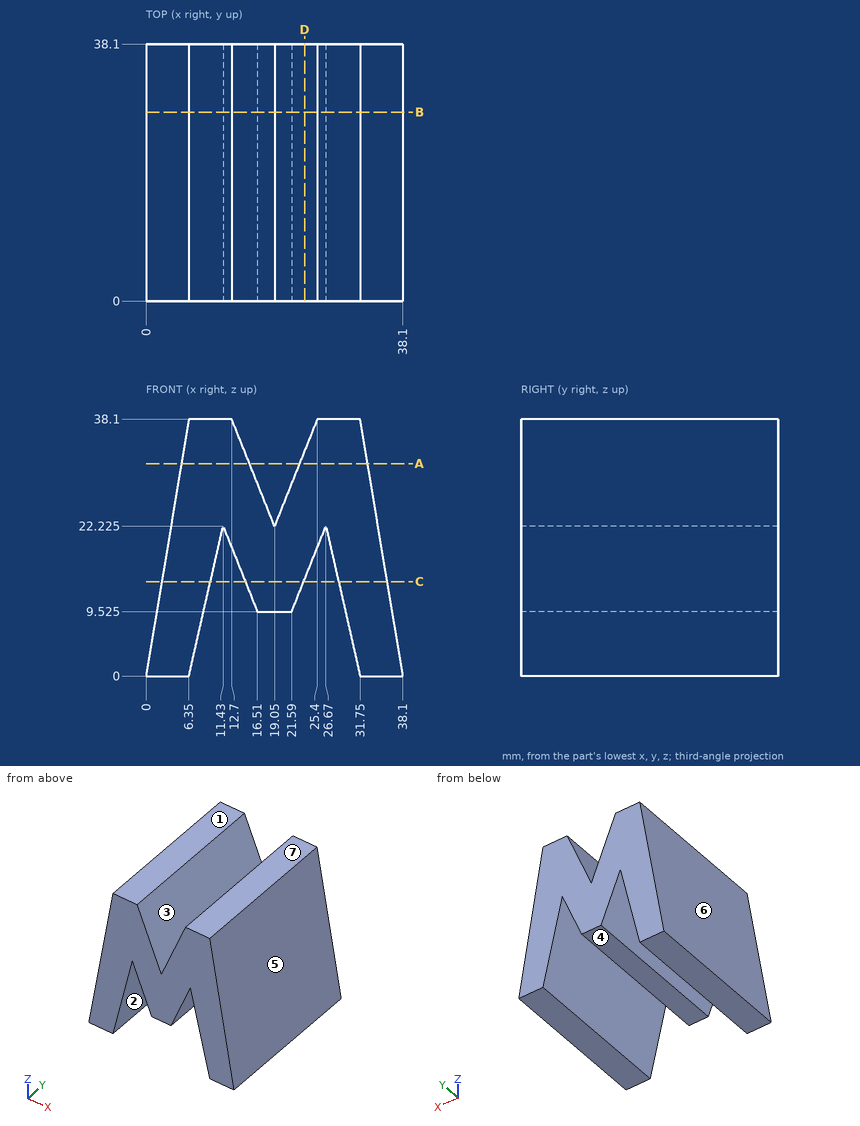
Here's the drawing with two shaded views (mm, measured from the low corner). I have some questions. A direction names the side the tool comes from. Coordinates: 2 decimals unless noted, no trailing zeros. Loops run counter-clockwise (first coordinate to the right, second up) from the corner with the lowest first, then second, coordinate; pieces in that order, holes last. Notation, with made-up numbers: M 62.5,61.5 L 104.5,61.5 A24 ccw 104.5,97.5 Z; hole C 75,-32 d11. An arc over 180 degrees is marked long. Return JSON: item names as keys, results as strings. Group by question number.
Item 1: Imagine slicing it at A-A (z = 31.5). Please give me the cut outline in (x, y).
Item 2: Imagine slicing it at C-C (z = 14). Please give me the cut outline in (x, y), and give its area (3 significant figures).
Item 3: Imagine slicing it at B-B (y = 28). Please give me the cut outline in (x, z) (3 decimals).
Item 4: On a 3-axis mill with a long thin cutter (end or side, diameter ignored), from which of +Z, -Z, +X, -X, +Y, -Y can I reach the whole of each face in a straight line? I mean the marked faces 1, 2 and 3. Say none if no direction works.
Item 5: Imagine slicing it at D-D (x = 23.5). Please give me the cut outline in (y, z), and give its area (3 significant figures).
Item 6: If I drill on L1, parallel to X at y = 34, z = 17; L2, parallel to X at y = 9.5, z = 20; L3, parallel to X at y = 10, z = 28, over which ranges is the centre line in solid material (lowest first)? Write a range as from..to.
Item 7: Thinking about a two-plate mould opening in X: for the marked faces 4, 5, 6 and 7, which applies, released by +X, released by -X, zero draft, split by the parting line, or undercut?
Item 8: I'm going to push flat-ended pins straight in: pin 1 Ø1 at (x, y) = (21, 19.5) entering from -Z (3 decimals); pin 2 Ø1 at (y, z) = (31, 22) entering from -X; pin 3 Ø8 at (y, z) = (8, 28.5) entering from +X. Where does each tip first touch, or does it pass through?
Verdict:
{
 "1": {"outline": "M 5.25,0 L 15.34,0 L 15.34,38.1 L 5.25,38.1 Z; M 22.76,0 L 32.85,0 L 32.85,38.1 L 22.76,38.1 Z"},
 "2": {"outline": "M 2.33,0 L 9.55,0 L 9.55,38.1 L 2.33,38.1 Z; M 14.72,0 L 23.38,0 L 23.38,38.1 L 14.72,38.1 Z; M 28.55,0 L 35.77,0 L 35.77,38.1 L 28.55,38.1 Z", "area": "880 mm^2"},
 "3": {"outline": "M 0,0 L 6.35,0 L 11.43,22.225 L 16.51,9.525 L 21.59,9.525 L 26.67,22.225 L 31.75,0 L 38.1,0 L 31.75,38.1 L 25.4,38.1 L 19.05,22.225 L 12.7,38.1 L 6.35,38.1 Z"},
 "4": {"face 1": "+Z, +X, -X, +Y, -Y", "face 2": "-Z, +Y, -Y", "face 3": "+Z, +Y, -Y"},
 "5": {"outline": "M 0,14.3 L 38.1,14.3 L 38.1,33.35 L 0,33.35 Z", "area": "726 mm^2"},
 "6": {"L1": "x = 2.83..10.24, 13.52..24.58, 27.86..35.27", "L2": "x = 3.33..10.92, 12.32..25.78, 27.18..34.77", "L3": "x = 4.67..16.74, 21.36..33.43"},
 "7": {"face 4": "undercut", "face 5": "released by +X", "face 6": "released by -X", "face 7": "zero draft"},
 "8": {"pin 1": "stops at z = 9.525", "pin 2": "stops at x = 3.58", "pin 3": "stops at x = 34.02"}
}
